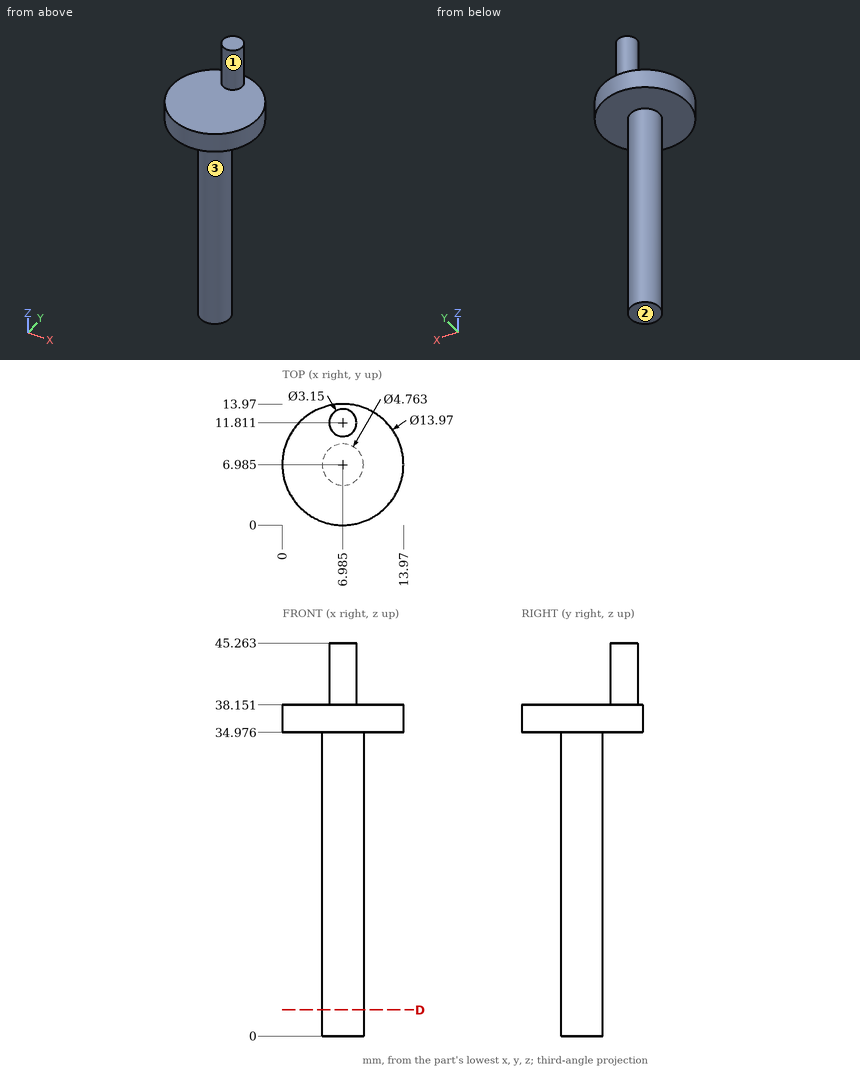
Study the drawing (mm; zero at the part's minimum x, y, z) and answer. A direction names the side the tool comes from. Give positions to 0.01 mm unless a question says otherwise; leave off trailing zeros. Order: outer loops, then holes, each group sorted by start corner. A loop starts at its lowest first (then second) coordinate and runs counter-clockwise, first axis right, second up. Notation, with made-up numbers: (77.5, 73) -> (81.5, 73) arc R33 cw to (81.5, 109) -> close; hole circle Ø11 at (71, 63.5). An arc over 180 degrees is marked (long way). Write item = value, one per line.
1. A cutting plane is placed at D-D, the plane z = 3. Write down the section's boundary in (x, y) (1 decimal), and give its area (3 significant figures).
Numbers:
outline = circle Ø4.8 at (7, 7)
area = 17.8 mm²
2. Given pin 1 (1 mm diameter, centred on x = 12.5, y = 9, fed in from +Z); pin 2 (4 mm diameter, centred on y = 11, z = 12.5, fed in from +X) (1 decimal); pin 3 (1.5 mm diameter, centred on y = 2, z = 23, fed in from +X); pin 4 (3 mm diameter, centred on x = 10, y = 12.5, fed in from -Z), each flat-ended and moving along its own axis, determine where each tip first touches the part or whether it passes through.
Numbers:
pin_1 = 38.15
pin_2 = 8.3
pin_3 = through
pin_4 = 34.98
3. For the marked faces 1, 2 and 3, determine the directions among +Z, -Z, +X, -X, +Y, -Y from which every point of the face is accessible in a straight line to the end or side of a thin tool.
Numbers:
face_1 = +Z
face_2 = -Z, +X, -X, +Y, -Y
face_3 = -Z
4. Straight lines are drawn through the part: line 1 along Z through (x, y) = (6.75, 5.75); line 2 along Z through (x, y) = (6.5, 10.5) (1 decimal); line 3 along X through (y, z) = (7.25, 33.5). For each, find the intervals that lie inside material, in ascending order.
Numbers:
line_1 = 0 to 38.15
line_2 = 35 to 45.3
line_3 = 4.62 to 9.35
